from build123d import *

# Parameters (mm, degrees)
ESQUISSE2_R             = 1.25
BOSS_EXTRU_1_DEPTH      = 130
ENL_V_MAT_EXTRU_1_DEPTH = 11


with BuildPart() as part:
    # Esquisse2 → Boss.-Extru.1 (new body)
    with BuildSketch(Plane.XY):
        Polygon((-1, -2), (1, -2), (3.383507185, -4), (1.5, -4), (1.5, -5), (5, -5), (5, -1.5), (4, -1.5), (4, -3.383507185), (2, -1), (2, 1), (4, 3.383507185), (4, 1.5), (5, 1.5), (5, 5), (1.5, 5), (1.5, 4), (3.383507185, 4), (1, 2), (-1, 2), (-3.383507185, 4), (-1.5, 4), (-1.5, 5), (-5, 5), (-5, 1.5), (-4, 1.5), (-4, 3.383507185), (-2, 1), (-2, -1), (-4, -3.383507185), (-4, -1.5), (-5, -1.5), (-5, -5), (-1.5, -5), (-1.5, -4), (-3.383507185, -4), align=None)
        Circle(ESQUISSE2_R, mode=Mode.SUBTRACT)
    extrude(amount=BOSS_EXTRU_1_DEPTH)

    # Esquisse3 → Enlèv. mat.-Extru.1 (cut, through all)
    with BuildSketch(Plane(origin=(0, 5, 0), x_dir=(1, 0, 0), z_dir=(0, 1, 0))):
        Polygon((-5, 0), (5, 0), (5, -10), align=None)
        Polygon((5, -125.857864376), (-5, -130), (5, -130), align=None)
    extrude(amount=-ENL_V_MAT_EXTRU_1_DEPTH, mode=Mode.SUBTRACT)


solid = part.part
The model under review builds one solid part; all positions refer to its coordinate system, in mm. A direction names the side the tool comes from. Give positions to 0.01 mm unless a question says otherwise; leave off trailing zeros.
1. For P1, Ø1.6, axis at y = 0, z = 51, coming from the -X side; P2, Ø5, axis at x = 0.5, z = 103.5, coming from the -Y side; P3, Ø1, axis at x = -3, y = -3, coming from the +Z side, all flat-tipped, find the tip position at first contact; note any pin that passes through.
2. Wall thickness on L1, parallel to Y at x = 0, z = 90.5; L2, parallel to Y at x = -2.25, z = 24.5: over which ranges is each line inside the solid? List them lowest first.
3. Draft analysis for pull direction Y (two halves, no side actions). For faces 1 (the flat face through (2.99, 2.18, 66.21)), 2 (the flat face through (3, -5, 66)), 3 (the flat face through (-5, 3, 64)), state which applies: +Y half, -Y half, draft (parallel to the pull), parting line (faces both ways), or undercut.
4. Tool access review of faces 4 (the flat face through (2, 0, 66)), 5 (the flat face through (0, -2, 65)), 6 (the flat face through (-5, -3, 64)), 7 (the flat face through (0, 2, 65)), 8 (the flat face through (-1.04, 1.18, 128.36)): name each direction out of +Z, -Z, +X, -X, +Y, -Y from which nothing blocks a thin tool from reaching the whole face with its end or side.
Worked answers:
1. P1: stops at x = -2
1. P2: stops at y = -5
1. P3: stops at z = 129.38
2. L1: y = -2 to -1.25, 1.25 to 2
2. L2: y = -5 to -4, -3.05 to -1.3, 1.3 to 3.05, 4 to 5
3. face 1: undercut
3. face 2: -Y half
3. face 3: draft
4. face 4: +Z, -Z, +X
4. face 5: +Z, -Z, -Y
4. face 6: +Z, -Z, -X, +Y, -Y
4. face 7: +Z, -Z, +Y
4. face 8: +Z, +X, +Y, -Y
